Geometry: see drawing. Coordinates: mm, zero at the bounding-box minimum. A direction names the side the tool comes from. Give positions to 0.01 mm unless a question says otherwise; leave off trailing zeros. Order: outer loops, then holes, each group sorted by start corner. A loop starts at its lowest first (then second) coordinate and runs counter-clockwise, first axis right, second up. Notation, with made-up numbers: (69, 40) - (101, 40) arc R23 ccw to (101, 64) - close; hole circle Ø7 at (42.25, -0.75). An arc over 180 degrees is marked (long way). Write each question's results on one line, items separated by ' | '. Start each with the question number.
Item 1: Section B-B on x = 8.75. Output: boundary loops of the cut face in (y, z).
Item 2: Section A-A on y = 2.5. Output: boundary loops of the cut face in (x, z).
Item 3: Mould query, pull axis Z, two halves, no side actions, for the marked faces 1, 2, 3 and 4. Classes: released by +Z, released by -Z, zero draft, split by the parting line, or undercut.
Item 4: Line query: line 1 along X through (y, z) = (4.25, 1.3); line 2 along X through (y, z) = (1.6, 3.3); line 3 along Y through (x, z) = (3.5, 2.6). Output: solid intervals per line, ascending.
Item 5: Contact query for flat-ended pins moving along their axis: pin 1 Ø1 at (x, z) = (5.5, 1.5) entering from +Y (1 decimal); pin 2 Ø2 at (x, y) = (7, 2) entering from +Z; pin 3 Ø1.3 at (y, z) = (2.5, 3) entering from -X. Output: stop coordinate, or through.
Item 6: Set-up query: the marked faces 5 and 6. Return all of +Z, -Z, +X, -X, +Y, -Y with unobstructed straight access to the full face (end or side cutting, diameter ignored); none if empty.
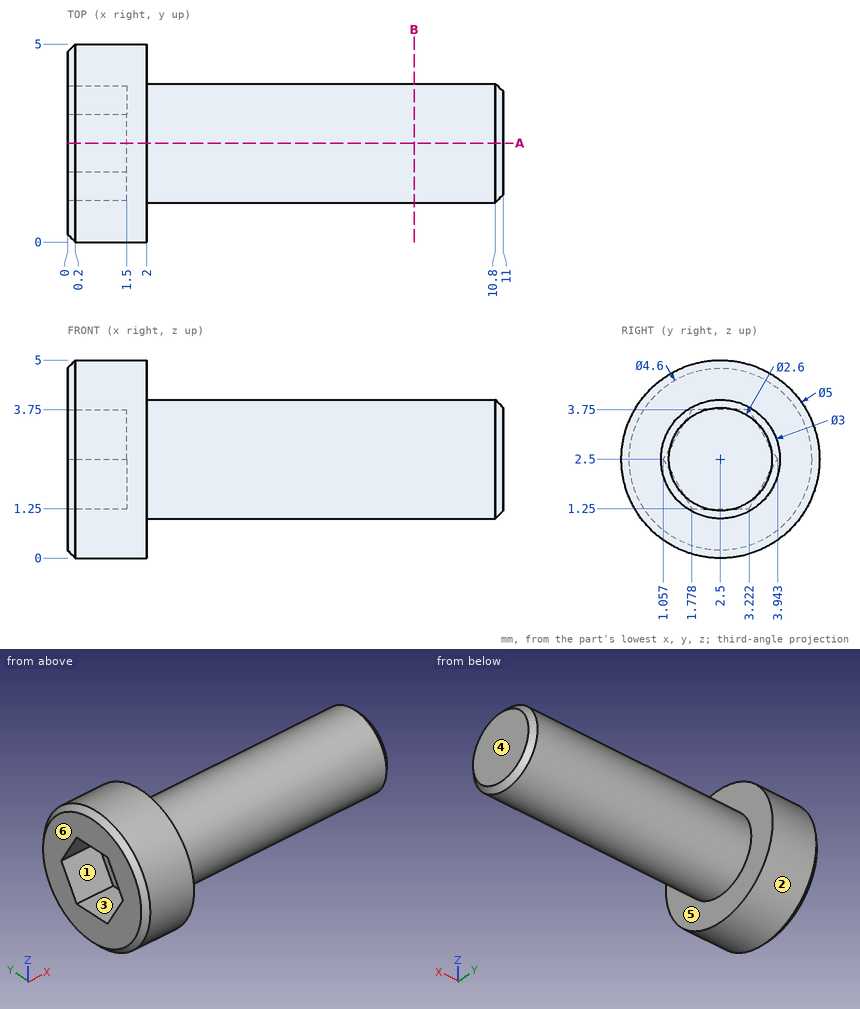
Evaluation:
1) outline: circle Ø3 at (2.5, 2.5)
2) outline: (0, 0.2) - (0.2, 0) - (2, 0) - (2, 1) - (10.8, 1) - (11, 1.2) - (11, 3.8) - (10.8, 4) - (2, 4) - (2, 5) - (0.2, 5) - (0, 4.8) - (0, 3.75) - (1.5, 3.75) - (1.5, 1.25) - (0, 1.25) - close
3) face 1: undercut | face 2: split by the parting line | face 3: undercut | face 4: zero draft
4) line 1: x = 0 to 2 | line 2: x = 1.5 to 11 | line 3: y = 1 to 4
5) pin 1: stops at y = 3.9 | pin 2: stops at z = 4 | pin 3: stops at x = 1.5
6) face 5: +X | face 6: +Z, -Z, -X, +Y, -Y
